Can you work these out from the model? Positions are in its coordinate system, mm. A direction names the side the tool comes from. Round coordinates to 2 decimals unless told otherwise and drop trailing zeros. Order: outer loops, then holes, each group sorted by start corner. A loop starts at its lowest first (then second) coordinate and runs counter-clockwise, first axis right, second up.
Q1. We'd pull the mould along X, two halves only. Please class faces 6 (the face through (9.14, -3.94, 9.1)), 7 (the face through (0, -4, -10)), 8 (the face through (-5.5, -2, 0)), 9 (the face through (-5.07, -1.92, 3.05)): pulls with the +X half, pulls with the -X half, needs draft (parallel to the pull), parting line crosses it, or undercut.
Q2. Will these pins go through, and if not, where does the flat tip stop? P1, Ø3, axis at y = 3, z = -2, coming from the +X side (3 decimals); P2, Ø2, axis at x = 1.5, y = 3, coming from the +Z side; P3, Ø1.2, axis at x = 1, y = 2.5, coming from the -Z side.
Q3. If we section it at A-A (z = 0.25): Please give me the cut outline in (x, y) (3 decimals).
Q4. If we section it at D-D (z = -4): Please give me the cut outline in (x, y) (3 decimals).
Q5. For faces 1 (the face through (0, 2, -4.65)), 2 (the face through (0, -2, -3.5)), 3 (the face through (-9.14, -3.94, -9.1)), 4 (the face through (-6.125, 2, 0)), 5 (the face through (0, 2, 4.65)), which set-ups out of +Z, -Z, +X, -X, +Y, -Y let a thin tool reach every point of the face, with its end or its side?
Q6. If we section it at C-C (x = -4.25): Please give me the cut outline in (y, z).
Q7. If we section it at B-B (y = -4.75): Please give me the cut outline in (x, z).
Q8. If I drill on line 1 (Z direction, x = -1.5, y = 3); line 2 (Z direction, x = -0.75, y = -7); line 3 (X direction, y = -7, z = -0.25), over which ranges is the centre line in solid material (lowest first)?
from build123d import *

# Parameters (mm, degrees)
F1_DEPTH = 8
F2_W     = 12.25
F2_H     = 9.3
F3_DEPTH = 4
F5_DEPTH = 25


with BuildPart() as f1:
    # F0 (on Front) → F1 (new body)
    with BuildSketch(Plane.XZ):
        with BuildLine():
            ThreePointArc((10, 7), (9.12132, 9.12132), (7, 10))
            Line((7, 10), (-7, 10))
            ThreePointArc((-7, 10), (-9.12132, 9.12132), (-10, 7))
            Line((-10, 7), (-10, -7))
            ThreePointArc((-10, -7), (-9.12132, -9.12132), (-7, -10))
            Line((-7, -10), (7, -10))
            ThreePointArc((7, -10), (9.12132, -9.12132), (10, -7))
            Line((10, -7), (10, 7))
        make_face()
    extrude(amount=F1_DEPTH)

    # F2 (on Front) → F3 (join)
    with BuildSketch(Plane.XZ):
        Rectangle(F2_W, F2_H)
    extrude(amount=-F3_DEPTH)

    # F4 (on face) → F5 (cut)
    with BuildSketch(Plane(origin=(0, 4, 0), x_dir=(-1, 0, 0), z_dir=(0, 1, 0))):
        with BuildLine():
            ThreePointArc((5.5, 2), (5.06066, 3.06066), (4, 3.5))
            Line((4, 3.5), (-4, 3.5))
            ThreePointArc((-4, 3.5), (-5.06066, 3.06066), (-5.5, 2))
            Line((-5.5, 2), (-5.5, -2))
            ThreePointArc((-5.5, -2), (-5.06066, -3.06066), (-4, -3.5))
            Line((-4, -3.5), (4, -3.5))
            ThreePointArc((4, -3.5), (5.06066, -3.06066), (5.5, -2))
            Line((5.5, -2), (5.5, 2))
        make_face()
    extrude(amount=-F5_DEPTH, mode=Mode.SUBTRACT)


solid = f1.part
Solution:
1. face 6: pulls with the +X half
1. face 7: needs draft
1. face 8: undercut
1. face 9: undercut
2. P1: stops at x = 6.125
2. P2: stops at z = 4.65
2. P3: stops at z = -4.65
3. outline: (-10, -8) - (-5.5, -8) - (-5.5, 4) - (-6.125, 4) - (-6.125, 0) - (-10, 0) - close; (5.5, -8) - (10, -8) - (10, 0) - (6.125, 0) - (6.125, 4) - (5.5, 4) - close
4. outline: (-10, -8) - (10, -8) - (10, 0) - (6.125, 0) - (6.125, 4) - (-6.125, 4) - (-6.125, 0) - (-10, 0) - close
5. face 1: -Z, +X, -X, +Y
5. face 2: +Y, -Y
5. face 3: -Z, -X, +Y, -Y
5. face 4: +Z, -Z, -X, +Y
5. face 5: +Z, +X, -X, +Y
6. outline: (-8, -10) - (0, -10) - (0, -4.65) - (4, -4.65) - (4, -3.48) - (-8, -3.48) - close; (-8, 3.48) - (4, 3.48) - (4, 4.65) - (0, 4.65) - (0, 10) - (-8, 10) - close
7. outline: (-10, -7) arc R3 ccw to (-7, -10) - (7, -10) arc R3 ccw to (10, -7) - (10, 7) arc R3 ccw to (7, 10) - (-7, 10) arc R3 ccw to (-10, 7) - close; hole (-5.5, -2) arc R1.5 ccw to (-4, -3.5) - (4, -3.5) arc R1.5 ccw to (5.5, -2) - (5.5, 2) arc R1.5 ccw to (4, 3.5) - (-4, 3.5) arc R1.5 ccw to (-5.5, 2) - close
8. line 1: z = -4.65 to -3.5, 3.5 to 4.65
8. line 2: z = -10 to -3.5, 3.5 to 10
8. line 3: x = -10 to -5.5, 5.5 to 10
